Source: CAD feature listing. Evaluate the final solid. Frame: model axes, mm. A direction names the side the tool comes from. Coordinates: 2 decimals unless noted, no trailing zeros. Loops run counter-clockwise (first coordinate to the right, second up) from the corner with the lowest first, then second, coordinate; pieces in that order, holes last. Notation, with made-up numbers: (-19, -23) -> (34, -23) arc R17 cw to (34, 4) -> close; hole circle Ø5 at (9.25, 11). An arc over 180 degrees is marked (long way). One line per question, with ' | ' between items. Start each with the question number.
```python
from build123d import *
from build123d.topology import SkipClean

# Parameters (mm, degrees)
SKETCH_1_R      = 5
EXTRUDE_1_DEPTH = 60
SKETCH_2_R      = 2.5
EXTRUDE_2_DEPTH = 20
FILLET_1_R      = 1


with BuildPart() as part:
    # 草图1 → 凸台-拉伸1 (new body)
    with BuildSketch(Plane(origin=(0, 0, 0), x_dir=(1, 0, 0), z_dir=(0, 1, 0))):
        with Locations(Location((0, 0, 0), (0, 0, 270))):
            Circle(SKETCH_1_R)
    extrude(amount=EXTRUDE_1_DEPTH)

    # 草图2 → 凸台-拉伸2 (add)
    with BuildSketch(Plane(origin=(0, 0, 0), x_dir=(1, 0, 0), z_dir=(0, 1, 0))):
        with Locations(Location((0, 0, 0), (0, 0, 270))):
            Circle(SKETCH_2_R)
    extrude(amount=-EXTRUDE_2_DEPTH)

    # 草图3 → 旋转1 (revolve)
    with SkipClean():  # the faces are left unmerged after this step: merging them gives an invalid solid
        with BuildSketch(Plane.XY):
            with BuildLine():
                ThreePointArc((2.5, -20), (1.767766953, -18.232233047), (0, -17.5))
                Line((0, -17.5), (0, -22.5))
                ThreePointArc((0, -22.5), (1.767766953, -21.767766953), (2.5, -20))
            make_face()
            with BuildLine():
                Line((0, -22.5), (0, -17.5))
                ThreePointArc((0, -17.5), (-2.5, -20), (0, -22.5))
            make_face()
        revolve(axis=Axis((0, -17.5, 0), (0, -1, 0)))

    # 圆角1
    fillet_1_edges = [part.edges().sort_by_distance(p)[0] for p in [
        (0, 0, -5),
        (0, 60, -5),
    ]]
    fillet(fillet_1_edges, radius=FILLET_1_R)


solid = part.part
```
(1) Access query for faces 1 (the flat face through (2, 0, 2)), 2 (the cylindrical face through (-4.88, 29.59, -1.08)). Directions: +Z, -Z, +X, -X, +Y, -Y. A direction counts if a zero-diameter tool reaches every point of the face in a straight line with its end or side. Return the directions, or none.
(2) Contact query for flat-ended pins moving along their axis: pin 1 Ø6 at (x, y) = (-2.5, -13.5) entering from -Z; pin 2 Ø1.5 at (x, z) = (-1, -2.5) entering from -Y; pin 3 Ø1.5 at (y, z) = (-7, 1) entering from +X. Output: stop coordinate, or through.
(3) Cut plane D-D, the plane y = 29.5. Return the cut outline in (x, z), and give its area (3 significant figures).
(4) Cut plane B-B, the plane z = 0. Return the cut outline in (x, y).
(5) Ray query, L1, parallel to Y at x = -2.75, z = -1.5; L2, parallel to X at y = -3.5, z = 0; L3, parallel to X at y = -9, z = -1.25. Return the intervals inside material, ascending.
(6) Cut plane A-A, the plane x = 0. Return the cut outline in (y, z), and give its area (3 significant figures).
(7) Cut plane C-C, the plane y = -14.5. Return the cut outline in (x, z).
Here are the results:
1) face 1: -Y | face 2: +Y, -Y
2) pin 1: stops at z = -2.5 | pin 2: stops at y = -21.57 | pin 3: stops at x = 2.49
3) outline: circle Ø10 at (0, 0) | area: 78.5 mm2
4) outline: (-5, 1) arc R1 ccw to (-4, 0) -> (-2.5, 0) -> (-2.5, -20) arc R2.5 ccw to (2.5, -20) -> (2.5, 0) -> (4, 0) arc R1 ccw to (5, 1) -> (5, 59) arc R1 ccw to (4, 60) -> (-4, 60) arc R1 ccw to (-5, 59) -> close
5) L1: y = 0 to 60 | L2: x = -2.5 to 2.5 | L3: x = -2.17 to 2.17
6) outline: (-20, -2.5) -> (0, -2.5) -> (0, -4) arc R1 ccw to (1, -5) -> (59, -5) arc R1 ccw to (60, -4) -> (60, 4) arc R1 ccw to (59, 5) -> (1, 5) arc R1 ccw to (0, 4) -> (0, 2.5) -> (-20, 2.5) arc R2.5 ccw to start | area: 709 mm2
7) outline: circle Ø5 at (0, 0)
